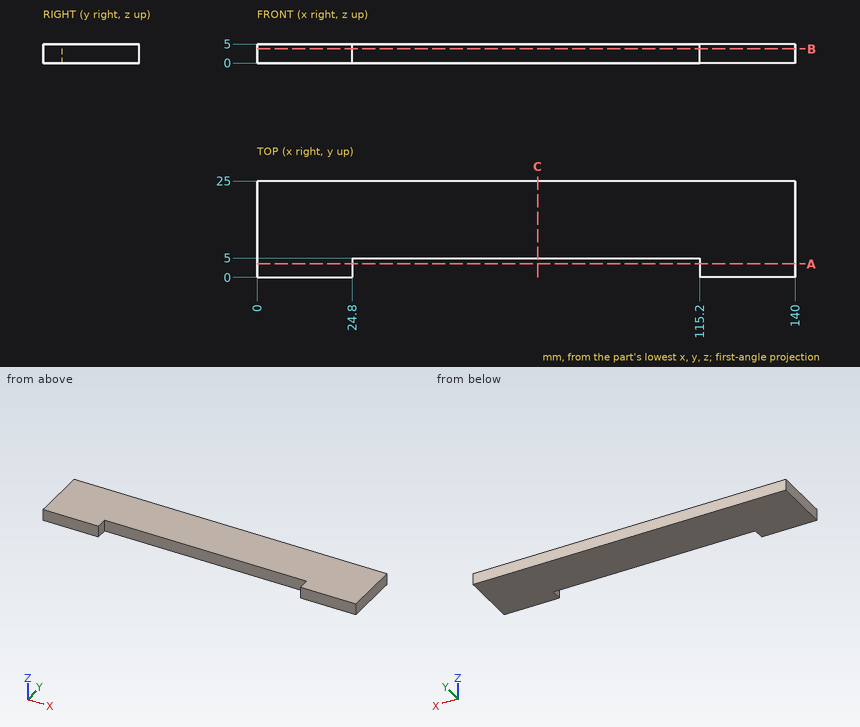
Design review of the part shown in the three views and the two pictorial views. Dimensions are in mm from the part's minimum x, y and z. Round coordinates to 2 decimals unless told otherwise and drop trailing zeros. Write each loop counter-clockwise with the first axis right and the second up, starting at its lowest first coordinate (ties: lowest second). Pieces come first, ordered by that corner, then holes.
Item 1: Wall thickness on L1, parallel to Y at x = 69.5, z = 3.8: over which ranges is the line inside the solid? List them lowest first.
Item 2: For pin 1 Ø2.5 at (x, z) = (92.5, 1.5) entering from -Y, flat-tipped, find the tip position at first contact; note if it passes through.
Item 3: Consider section A-A on y = 3.5. Give the boundary of the cut face in (x, z), and give its area (3 significant figures).
Item 4: Consider section C-C on x = 73. Give the boundary of the cut face in (y, z), and give its area (3 significant figures).
Item 5: Consider section B-B on z = 3.7. Give the boundary of the cut face in (x, y), and give its area (3 significant figures).
Check values:
1. L1: y = 5 to 25
2. pin 1: stops at y = 5
3. outline: (0, 0) - (24.8, 0) - (24.8, 5) - (0, 5) - close; (115.2, 0) - (140, 0) - (140, 5) - (115.2, 5) - close
3. area: 248 mm2
4. outline: (5, 0) - (25, 0) - (25, 5) - (5, 5) - close
4. area: 100 mm2
5. outline: (0, 0) - (24.8, 0) - (24.8, 5) - (115.2, 5) - (115.2, 0) - (140, 0) - (140, 25) - (0, 25) - close
5. area: 3,050 mm2
